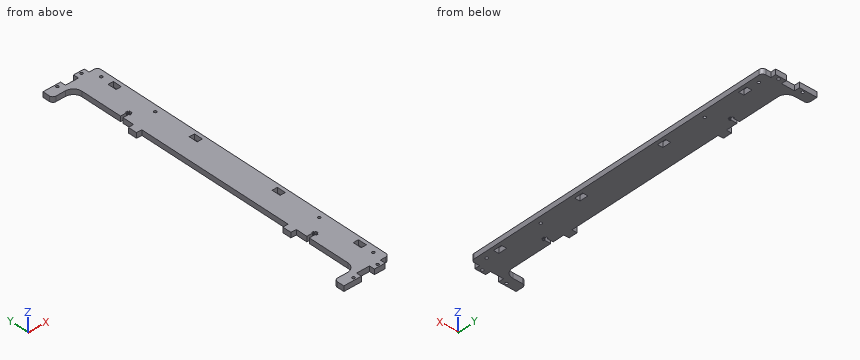
from build123d import *

# Parameters (mm, degrees)
SKETCH_1_R      = 1.55
SKETCH_1_W      = 6.1
SKETCH_1_H      = 10
EXTRUDE_1_DEPTH = 6


with BuildPart() as part:
    # Эскиз1 → Бобышка-Вытянуть1 (new body)
    with BuildSketch(Plane.XY):
        with BuildLine():
            Line((2.8, 115.55), (2.8, 114.35))
            Line((2.8, 114.35), (5, 114.35))
            Line((5, 114.35), (5, 115.55))
            Line((5, 115.55), (6.5, 115.55))
            Line((6.5, 115.55), (6.5, 118.65))
            Line((6.5, 118.65), (5, 118.65))
            Line((5, 118.65), (5, 119.85))
            Line((5, 119.85), (2.8, 119.85))
            Line((2.8, 119.85), (2.8, 118.65))
            Line((2.8, 118.65), (-4, 118.65))
            Line((-4, 118.65), (-4, 167.1))
            ThreePointArc((-4, 167.1), (-6.928932188, 174.171067812), (-14, 177.1))
            Line((-14, 177.1), (-25, 177.1))
            ThreePointArc((-25, 177.1), (-27.828427125, 178.271572875), (-29, 181.1))
            Line((-29, 181.1), (-29, 189.1))
            Line((-29, 189.1), (-8.55, 189.1))
            Line((-8.55, 189.1), (-8.55, 183))
            Line((-8.55, 183), (6.55, 183))
            Line((6.55, 183), (6.55, 189.1))
            Line((6.55, 189.1), (19, 189.1))
            Line((19, 189.1), (19, 183.1))
            Line((19, 183.1), (25, 183.1))
            ThreePointArc((25, 183.1), (27.828427125, 181.928427125), (29, 179.1))
            Line((29, 179.1), (29, -179.1))
            ThreePointArc((29, -179.1), (27.828427125, -181.928427125), (25, -183.1))
            Line((25, -183.1), (19, -183.1))
            Line((19, -183.1), (19, -189.1))
            Line((19, -189.1), (6.55, -189.1))
            Line((6.55, -189.1), (6.55, -183))
            Line((6.55, -183), (-8.55, -183))
            Line((-8.55, -183), (-8.55, -189.1))
            Line((-8.55, -189.1), (-29, -189.1))
            Line((-29, -189.1), (-29, -181.1))
            ThreePointArc((-29, -181.1), (-27.828427125, -178.271572875), (-25, -177.1))
            Line((-25, -177.1), (-14, -177.1))
            ThreePointArc((-14, -177.1), (-6.928932188, -174.171067812), (-4, -167.1))
            Line((-4, -167.1), (-4, -118.65))
            Line((-4, -118.65), (2.8, -118.65))
            Line((2.8, -118.65), (2.8, -119.85))
            Line((2.8, -119.85), (5, -119.85))
            Line((5, -119.85), (5, -118.65))
            Line((5, -118.65), (6.5, -118.65))
            Line((6.5, -118.65), (6.5, -115.55))
            Line((6.5, -115.55), (5, -115.55))
            Line((5, -115.55), (5, -114.35))
            Line((5, -114.35), (2.8, -114.35))
            Line((2.8, -114.35), (2.8, -115.55))
            Line((2.8, -115.55), (-4, -115.55))
            Line((-4, -115.55), (-4, -102.35))
            Line((-4, -102.35), (-10.1, -102.1))
            Line((-10.1, -102.1), (-10.1, -92.1))
            Line((-10.1, -92.1), (-4, -91.85))
            Line((-4, -91.85), (-4, 91.85))
            Line((-4, 91.85), (-10.1, 92.1))
            Line((-10.1, 92.1), (-10.1, 102.1))
            Line((-10.1, 102.1), (-4, 102.35))
            Line((-4, 102.35), (-4, 115.55))
            Line((-4, 115.55), (2.8, 115.55))
        make_face()
        with Locations((-15, 186.1)):
            Circle(SKETCH_1_R, mode=Mode.SUBTRACT)
        with Locations((13, 186.1)):
            Circle(SKETCH_1_R, mode=Mode.SUBTRACT)
        with Locations((22, 103.1)):
            Circle(SKETCH_1_R, mode=Mode.SUBTRACT)
        with Locations((22, 171.1)):
            Circle(SKETCH_1_R, mode=Mode.SUBTRACT)
        with Locations((-15, -186.1)):
            Circle(SKETCH_1_R, mode=Mode.SUBTRACT)
        with Locations((13, -186.1)):
            Circle(SKETCH_1_R, mode=Mode.SUBTRACT)
        with Locations((22, -103.1)):
            Circle(SKETCH_1_R, mode=Mode.SUBTRACT)
        with Locations((22, -171.1)):
            Circle(SKETCH_1_R, mode=Mode.SUBTRACT)
        with Locations((22, 154.1)):
            Rectangle(SKETCH_1_W, SKETCH_1_H, mode=Mode.SUBTRACT)
        with Locations((22, 52.1)):
            Rectangle(SKETCH_1_W, SKETCH_1_H, mode=Mode.SUBTRACT)
        with Locations((22, -154.1)):
            Rectangle(SKETCH_1_W, SKETCH_1_H, mode=Mode.SUBTRACT)
        with Locations((22, -52.1)):
            Rectangle(SKETCH_1_W, SKETCH_1_H, mode=Mode.SUBTRACT)
    extrude(amount=EXTRUDE_1_DEPTH)


solid = part.part
Could you check a few things on this model? Use its own coordinates, in mm. Coordinates: 2 decimals unless noted, no trailing zeros. Loops run counter-clockwise (first coordinate to the right, second up) from the corner with the lowest first, then second, coordinate; pieces in that order, holes last.
1. For P1, Ø3, axis at x = 2, z = 4, coming from the +Y side; P2, Ø3, axis at y = 154, z = 4, coming from the -X side; P3, Ø2, axis at x = 1.5, z = 3.5, coming from the -Y side, each with a flat end and sliding along its axis, tell me the tip position at first contact or that it passes through.
2. I need wall thicknesses on L1, parallel to Y at x = -15, z = 2.4; L2, parallel to Y at x = -3, z = 4.55; L3, parallel to X at y = 186.1, z = 4.6. Which ranges of each line are inside material? Lowest first, please.
3. Imagine slicing it at B-B (z = 2.35). Give the number of separate pieces and of enclosed holes in the cut face, and give its area (3 significant figures).
4. Imagine slicing it at A-A (y = -72.5). Please give me the cut outline in (x, z).
Computed values:
1. P1: stops at y = 183
1. P2: stops at x = -4
1. P3: stops at y = -183
2. L1: y = -189.1 to -187.65, -184.55 to -177.1, 177.1 to 184.55, 187.65 to 189.1
2. L2: y = -183 to -118.65, -115.55 to 115.55, 118.65 to 183
2. L3: x = -29 to -16.55, -13.45 to -8.55, 6.55 to 11.45, 14.55 to 19
3. separate pieces: 1
3. enclosed holes: 12
3. area: 12,600 mm2
4. outline: (-4, 0) - (29, 0) - (29, 6) - (-4, 6) - close
